Design review of the part built by this model. Coordinates are the model's own, in mm. Face numbers are marked on the shaded views. A direction names the side the tool comes from. Coordinates: 2 decimals unless noted, no trailing zeros. Write each loop counter-clockwise with the first axis right and the second up, starting at its lowest first coordinate (ties: lowest second). Pieces come first, ordered by that corner, then holes. Notation, with made-up numbers: (-21, 79) - (-2, 79) arc R17 ccw to (-2, 99) - close; hole circle Ø10 at (73.25, 23.5). An arc over 180 degrees is marked (long way). One line per item, written item: value.
from build123d import *

# Parameters (mm, degrees)
F1_DEPTH = 6


with BuildPart() as f1:
    # F0 (on Right) → F1 (new body)
    with BuildSketch(Plane.YZ):
        with BuildLine():
            Line((3.4, 48), (0, 48))
            Line((0, 48), (0, 0))
            Line((0, 0), (3.4, 0))
            Line((3.4, 0), (3.4, 3.75))
            Line((3.4, 3.75), (2.2, 3.75))
            Line((2.2, 3.75), (2.2, 6.25))
            Line((2.2, 6.25), (3.4, 6.25))
            Line((3.4, 6.25), (3.4, 10))
            Line((3.4, 10), (5, 10))
            Line((5, 10), (6.6, 10))
            Line((6.6, 10), (6.6, 6.25))
            Line((6.6, 6.25), (7.8, 6.25))
            Line((7.8, 6.25), (7.8, 3.75))
            Line((7.8, 3.75), (6.6, 3.75))
            Line((6.6, 3.75), (6.6, 0))
            Line((6.6, 0), (10, 0))
            Line((10, 0), (10, -6))
            Line((10, -6), (20, -6))
            Line((20, -6), (20, 0))
            ThreePointArc((20, 0), (12.928932, 2.928932), (10, 10))
            Line((10, 10), (10, 38))
            ThreePointArc((10, 38), (12.928932, 45.071068), (20, 48))
            Line((20, 48), (20, 54))
            Line((20, 54), (10, 54))
            Line((10, 54), (10, 48))
            Line((10, 48), (6.6, 48))
            Line((6.6, 48), (6.6, 44.25))
            Line((6.6, 44.25), (7.8, 44.25))
            Line((7.8, 44.25), (7.8, 41.75))
            Line((7.8, 41.75), (6.6, 41.75))
            Line((6.6, 41.75), (6.6, 38))
            Line((6.6, 38), (5, 38))
            Line((5, 38), (3.4, 38))
            Line((3.4, 38), (3.4, 41.75))
            Line((3.4, 41.75), (2.2, 41.75))
            Line((2.2, 41.75), (2.2, 44.25))
            Line((2.2, 44.25), (3.4, 44.25))
            Line((3.4, 44.25), (3.4, 48))
        make_face()
    extrude(amount=F1_DEPTH)


solid = f1.part
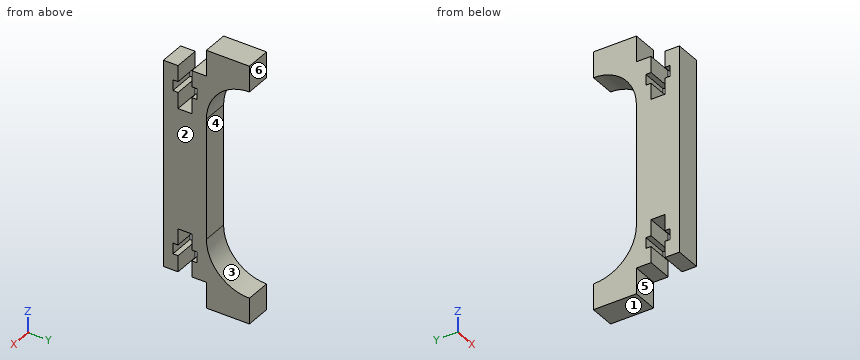
1. For the marked faces 4, 5 and 6, list the 3-axis set-ups (+Z, -Z, +X, -X, +Y, -Y) from which the entire face can be reached by the end or side of a thin tool; tool diameter is ignored.
Answer block:
face 4: +X, -X, +Y
face 5: -Z, +X, -X, -Y
face 6: +Z, -Z, +X, -X, +Y
2. Consider section D-D, the plane y = 1.5. Write out the cut boundary in (x, z).
Answer block:
outline: (0, 0) - (6, 0) - (6, 48) - (0, 48) - close
3. Insertion check: pin 1 Ø1.1 at (x, z) = (3.5, 39.5) entering from -Y; pin 2 Ø1 at (x, y) = (3.5, 2.5) entering from +Z; pin 3 Ø0.6 at (x, y) = (3, 3) entering from -Z; pin 4 Ø1.1 at (x, z) = (2, 7.5) entering from +Y. Each pin has a flat end and moves straight along its axis. Give the tip position at first contact, or say it passes through.
Answer block:
pin 1: stops at y = 0
pin 2: stops at z = 48
pin 3: stops at z = 0
pin 4: stops at y = 10.48
4. Consider section B-B, the plane z = 41. Write out the cut boundary in (x, y), then the cut area to 3 significant figures.
Answer block:
outline: (0, 0) - (6, 0) - (6, 3.4) - (0, 3.4) - close; (0, 6.6) - (6, 6.6) - (6, 10.46) - (0, 10.46) - close
area: 43.6 mm^2
5. Consider section C-C, the plane z = 31. Write out the cut boundary in (x, y), then the cut area to 3 significant figures.
Answer block:
outline: (0, 0) - (6, 0) - (6, 10) - (0, 10) - close
area: 60.0 mm^2
6. Consider section A-A, the plane y = 11. Write out the cut boundary in (x, z), then the cut area to 3 significant figures.
Answer block:
outline: (0, -6) - (6, -6) - (6, 5.64) - (0, 5.64) - close; (0, 42.36) - (6, 42.36) - (6, 54) - (0, 54) - close
area: 140 mm^2
7. Mouldability with a two-part tool opening along Z and no side actions: class the marked faces 1, 2 and 3 as released by +Z, released by -Z, zero draft, split by the parting line, or undercut.
Answer block:
face 1: released by -Z
face 2: zero draft
face 3: undercut
8. Wall thickness on line 1 along Z through (x, y) = (4.05, 3); line 2 along Y through (x, z) = (2.7, -3); line 3 along Z through (x, y) = (4.5, 12): over which ranges is each line inside the solid? List them lowest first.
Answer block:
line 1: z = 0 to 3.75, 6.25 to 41.75, 44.25 to 48
line 2: y = 10 to 20
line 3: z = -6 to 4, 44 to 54
